Source: CAD feature listing. Evaluate the final solid. Frame: model axes, mm. Face numbers are marked on the shaded views. A direction names the side the tool comes from. Give positions to 0.01 mm unless a question says otherwise; leave off trailing zeros. Write each loop counter-clockwise with the first axis right and the second up, starting at its lowest first coordinate (ties: lowest second). Pieces come first, ordered by that corner, then holes. Notation, with made-up numbers: (-4, 38) - (32, 38) arc R23 cw to (32, 55) - close; hole circle Ø9 at (-38.5, 7.5). An arc over 180 degrees is marked (long way). Answer as a JSON object with one key per item and string values. Group by question number.
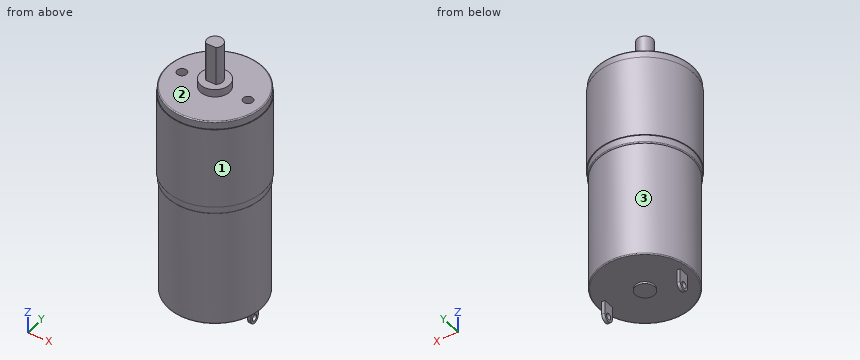
from build123d import *

# Parameters (mm, degrees)
SKETCH1_R                       = 12.3
BOSS_EXTRUDE1_DEPTH             = 2
FILLET1_R                       = 0.25
SKETCH3_R                       = 12.5
BOSS_EXTRUDE3_DEPTH             = 21
SKETCH4_R                       = 12.3
BOSS_EXTRUDE4_DEPTH             = 2
FILLET3_R                       = 0.25
SKETCH5_R                       = 12.05
BOSS_EXTRUDE5_DEPTH             = 30
FILLET4_R                       = 0.25
SKETCH6_W                       = 0.807133711
SKETCH6_H                       = 2.824967988
BOSS_EXTRUDE6_DEPTH             = 5
SKETCH7_R                       = 0.8
CUT_EXTRUDE1_DEPTH              = 23.589171386
SKETCH8_R                       = 2.5
BOSS_EXTRUDE7_DEPTH             = 0.5
SKETCH9_R                       = 3.75
BOSS_EXTRUDE8_DEPTH             = 2
BOSS_EXTRUDE9_DEPTH             = 10
TAP_DRILL_FOR_M3X0_5_TAP1_D     = 2.5
TAP_DRILL_FOR_M3X0_5_TAP1_DEPTH = 10


with BuildPart() as part:
    # Sketch1 → Boss-Extrude1 (new body)
    with BuildSketch(Plane.XY):
        Circle(SKETCH1_R)
    extrude(amount=BOSS_EXTRUDE1_DEPTH)

    # Fillet1
    fillet1_edges = [part.edges().sort_by_distance(p)[0] for p in [
        (-12.3, 0, 2),
    ]]
    fillet(fillet1_edges, radius=FILLET1_R)

    # Sketch3 → Boss-Extrude3 (add)
    with BuildSketch(Plane(origin=(0, 0, 0), x_dir=(-1, 0, 0), z_dir=(0, 0, -1))):
        Circle(SKETCH3_R)
    extrude(amount=BOSS_EXTRUDE3_DEPTH)

    # Sketch4 → Boss-Extrude4 (add)
    with BuildSketch(Plane(origin=(0, 0, -21), x_dir=(-1, 0, 0), z_dir=(0, 0, -1))):
        Circle(SKETCH4_R)
    extrude(amount=BOSS_EXTRUDE4_DEPTH)

    # Fillet3
    fillet3_edges = [part.edges().sort_by_distance(p)[0] for p in [
        (12.3, 0, -23),
    ]]
    fillet(fillet3_edges, radius=FILLET3_R)

    # Sketch5 → Boss-Extrude5 (add)
    with BuildSketch(Plane(origin=(0, 0, -23), x_dir=(-1, 0, 0), z_dir=(0, 0, -1))):
        Circle(SKETCH5_R)
    extrude(amount=BOSS_EXTRUDE5_DEPTH)

    # Fillet4
    fillet4_edges = [part.edges().sort_by_distance(p)[0] for p in [
        (12.05, 0, -53),
    ]]
    fillet(fillet4_edges, radius=FILLET4_R)

    # Sketch6 → Boss-Extrude6 (add)
    with BuildSketch(Plane(origin=(0, 0, -53), x_dir=(-1, 0, 0), z_dir=(0, 0, -1))):
        with Locations((-9.685604531, 0.126114642)):
            Rectangle(SKETCH6_W, SKETCH6_H)
        with Locations((9.685604531, 0.126114642)):
            Rectangle(SKETCH6_W, SKETCH6_H)
    extrude(amount=BOSS_EXTRUDE6_DEPTH)

    # Sketch7 → Cut-Extrude1 (cut, through all)
    with BuildSketch(Plane(origin=(10.089171386, 0, 0), x_dir=(0, 0, -1), z_dir=(1, 0, 0))):
        with Locations((56.439265275, 0.126114642)):
            Circle(SKETCH7_R)
        with BuildLine():
            Line((56.439265275, 1.538598636), (58, 1.538598636))
            Line((58, 1.538598636), (58, -1.286369352))
            Line((58, -1.286369352), (56.439265275, -1.286369352))
            ThreePointArc((56.439265275, -1.286369352), (57.851749269, 0.126114642), (56.439265275, 1.538598636))
        make_face()
    extrude(amount=-CUT_EXTRUDE1_DEPTH, mode=Mode.SUBTRACT)

    # Sketch8 → Boss-Extrude7 (add)
    with BuildSketch(Plane(origin=(0, 0, -53), x_dir=(-1, 0, 0), z_dir=(0, 0, -1))):
        Circle(SKETCH8_R)
    extrude(amount=BOSS_EXTRUDE7_DEPTH)

    # Sketch9 → Boss-Extrude8 (add)
    with BuildSketch(Plane.XY.offset(2)):
        Circle(SKETCH9_R)
    extrude(amount=BOSS_EXTRUDE8_DEPTH)

    # Sketch10 → Boss-Extrude9 (add)
    with BuildSketch(Plane.XY.offset(4)):
        with BuildLine():
            Line((-1.288271492, -1.529822396), (1.262174935, -1.551423357))
            ThreePointArc((1.262174935, -1.551423357), (0.016938357, 1.999928272), (-1.288271492, -1.529822396))
        make_face()
    extrude(amount=BOSS_EXTRUDE9_DEPTH)

    # Tap Drill for M3x0.5 Tap1
    with Locations(Plane.XY.offset(2)):
        with Locations((8.5, 0), (-8.5, 0)):
            Hole(TAP_DRILL_FOR_M3X0_5_TAP1_D / 2, depth=TAP_DRILL_FOR_M3X0_5_TAP1_DEPTH)


solid = part.part
Q1. Section C-C on z = -11. Return the cut outline in (x, y), then the cut area to 3 significant figures.
Q2. First-contact query: pin 1 Ø12 at (x, z) = (-9.5, -18.5) entering from -Y; pin 2 Ø1 at (x, y) = (7.5, 0) entering from -Z; pin 3 Ø10 at (x, y) = (-3, 2) entering from -Z. Flat tips, straight axial feed; report the tip coordinate or a pass-through.
Q3. Ray query, probe 1 along Z at (x, y) = (-1, 9); probe 2 along Y at (x, z) = (8.5, -2); probe 3 along Z at (x, y) = (-0.25, 0.25). Return the intervals inside material, ascending. Write a range as [from, to].
Q4. Section A-A on z = -42. Return the cut outline in (x, y), then the cut area to 3 significant figures.
Q5. Reachability of the marked faces 1, 2 and 3 from +Z, -Z, +X, -X, +Y, -Y: full face, straight path, thin tool, end or side. Return the list, or none.
Taken from the geometry:
{
 "1": {"outline": "circle Ø25 at (0, 0)", "area": "491 mm²"},
 "2": {"pin 1": "stops at y = -12", "pin 2": "stops at z = -53", "pin 3": "stops at z = -53.5"},
 "3": {"probe 1": "z = [-53, 2]", "probe 2": "y = [-9.17, -1.25], [1.25, 9.17]", "probe 3": "z = [-53.5, 14]"},
 "4": {"outline": "circle Ø24.1 at (0, 0)", "area": "456 mm²"},
 "5": {"face 1": "+Z, -Z", "face 2": "+Z", "face 3": "-Z"}
}
